Source: three-view drawing plus pictorial views. Frame: mm from the lowest corner of the part. Give positions to 0.01 mm unless a question says otherwise; leave off trailing zeros. Order: outer loops, then holes, each group sorted by start corner. A loop starts at its lowest first (then second) coordinate and runs counter-clockwise, first axis right, second up. Notation, with made-up numbers: (4.25, 73) - (22.25, 73) arc R22 ccw to (22.25, 95) - close; hole circle Ø6 at (53.25, -8.5). An arc over 180 degrees is marked (long way). Use CSV: the item, a comma, the result in double quotes.
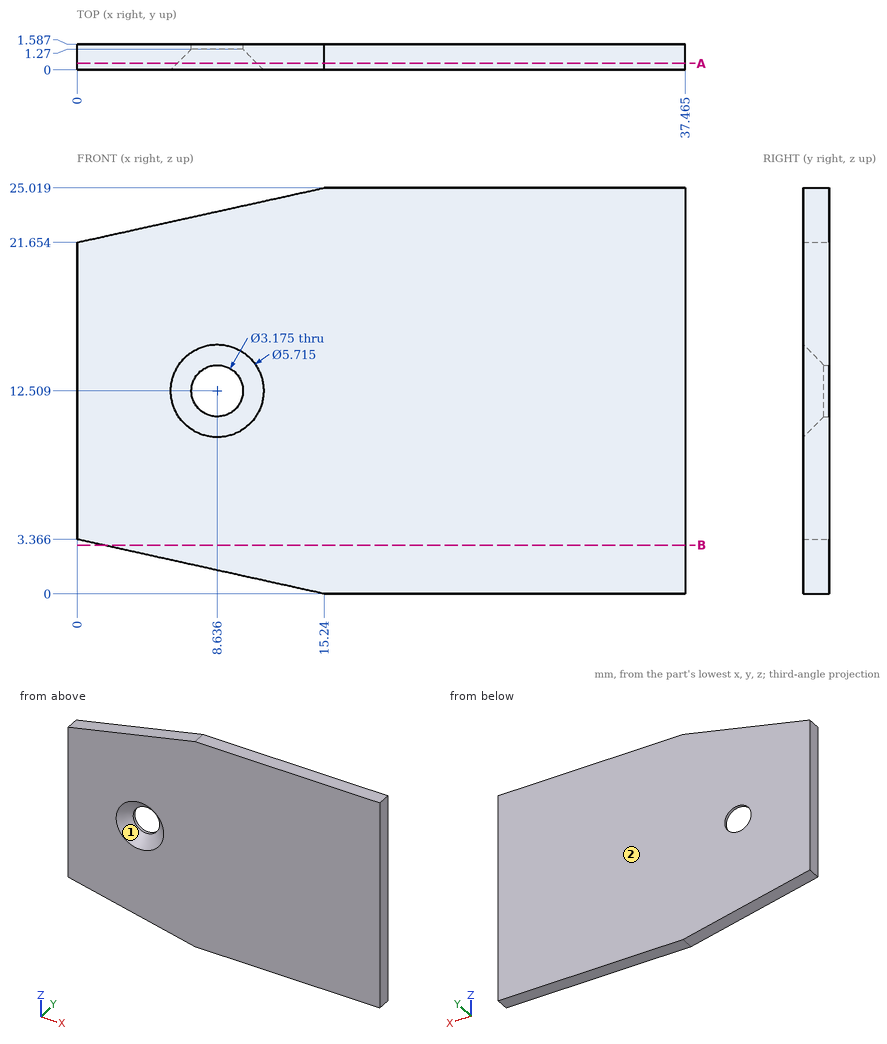
Item 1: Mould query, pull axis Z, two halves, no side actions, for the marked faces 1 and 2. Classes: released by +Z, released by -Z, zero draft, split by the parting line, or undercut.
Filled in:
face 1,"undercut"
face 2,"zero draft"
Item 2: First-contact query: pin 1 (3.5 mm diameter, centred on x = 8.64, z = 12.51, fed in from +Y). Flat tip, straight axial feed; report the tip coordinate or a pass-through.
Filled in:
pin 1,"stops at y = 1.59"
Item 3: Section B-B on z = 3. Return the cut outline in (x, y) (1 decimal).
Filled in:
outline,"(1.7, 0) - (37.5, 0) - (37.5, 1.6) - (1.7, 1.6) - close"
Item 4: Material intervals for line 1 (X direction, y = 0.35, z = 10.5) (1 decimal); line 2 (X direction, y = 1.15, z = 13.75) (1 decimal); line 3 (Z direction, x = 15, y = 0.55) (1 decimal), sorted ascending. Write a range as from..to.
Filled in:
line 1,"x = 0..7.1, 10.1..37.5"
line 2,"x = 0..7.5, 9.8..37.5"
line 3,"z = 0.1..25"
Item 5: Section A-A on y = 0.4. Return the cut outline in (x, z) (1 decimal), then the cut area to 3 significant figures.
Filled in:
outline,"(0, 3.4) - (15.2, 0) - (37.5, 0) - (37.5, 25) - (15.2, 25) - (0, 21.7) - close; hole circle Ø4.9 at (8.6, 12.5)"
area,"867 mm2"
